Model file for the job. Use its own axes, mm. A direction names the side the tool comes from. Round coordinates to 2 decimals unless told otherwise and drop trailing zeros. Loops run counter-clockwise (first coordinate to the right, second up) from the corner with the lowest first, then second, coordinate; pieces in that order, holes last. Notation, with made-up numbers: M 67,20 L 108,20 A23 cw 108,37 Z; hole C -27,-18 d1. An arc over 180 degrees is marked long. Answer in a Markdown table with one row per item.
from build123d import *
from build123d.topology import SkipClean

# Parameters (mm, degrees)
SKETCH2_W                = 120
SKETCH2_H                = 250
BOSS_EXTRUDE1_DEPTH      = 50
CUT_EXTRUDE1_DEPTH       = 295.78805946
CUT_EXTRUDE1_DEPTH_BACK  = 295.78805946
CUT_EXTRUDE2_DEPTH       = 100
CUT_EXTRUDE3_DEPTH       = 282.780056072
CUT_EXTRUDE3_DEPTH_BACK  = 282.780056072
FILLET1_R                = 25
CUT_EXTRUDE5_DEPTH       = 60
FILLET4_R                = 12
SKETCH8_R                = 25
BOSS_EXTRUDE2_DEPTH      = 150.7
CUT_EXTRUDE11_DEPTH      = 422.260596306
CUT_EXTRUDE11_DEPTH_BACK = 422.260596306
SKETCH9_R                = 25


with BuildPart() as part:
    # Sketch2 → Boss-Extrude1 (new, symmetric)
    with BuildSketch(Plane(origin=(0, 0, 0), x_dir=(1, 0, 0), z_dir=(0, 1, 0))):
        with Locations((-60, 125)):
            Rectangle(SKETCH2_W, SKETCH2_H)
    extrude(amount=BOSS_EXTRUDE1_DEPTH, both=True)

    # Sketch3 → Cut-Extrude1 (cut, two sides: drawn at the far end of the back side and taken through both)
    with BuildSketch(Plane(origin=(0, 50, 0), x_dir=(1, 0, 0), z_dir=(0, 1, 0)).offset(-CUT_EXTRUDE1_DEPTH_BACK)):
        with BuildLine():
            Line((-120, 250), (-120, 104))
            ThreePointArc((-120, 104), (-115.759222637, 126.156468376), (-103.636363636, 145.180915101))
            ThreePointArc((-103.636363636, 145.180915101), (-93.533981136, 161.034620706), (-90, 179.498344353))
            Line((-90, 179.498344353), (-90, 250))
            Line((-90, 250), (-120, 250))
        make_face()
        with BuildLine():
            ThreePointArc((-16.363636364, 145.180915101), (-4.240777363, 126.156468376), (0, 104))
            Line((0, 104), (0, 250))
            Line((0, 250), (-30, 250))
            Line((-30, 250), (-30, 179.498344353))
            ThreePointArc((-30, 179.498344353), (-26.466018864, 161.034620706), (-16.363636364, 145.180915101))
        make_face()
        with BuildLine():
            ThreePointArc((-30, 100), (-38.786796564, 121.213203436), (-60, 130))
            Line((-60, 130), (-60, 0))
            Line((-60, 0), (-30, 0))
            Line((-30, 0), (-30, 100))
        make_face()
        with BuildLine():
            Line((-60, 0), (-60, 130))
            ThreePointArc((-60, 130), (-81.213203436, 121.213203436), (-90, 100))
            Line((-90, 100), (-90, 0))
            Line((-90, 0), (-60, 0))
        make_face()
    extrude(amount=CUT_EXTRUDE1_DEPTH + CUT_EXTRUDE1_DEPTH_BACK, mode=Mode.SUBTRACT)

    # Sketch4 → Cut-Extrude2 (cut)
    with BuildSketch(Plane(origin=(0, 0, 0), x_dir=(0, 0, -1), z_dir=(1, 0, 0))):
        Polygon((104, 50), (104, 29.703239367), (250, 29.703239367), (250, 50), (179.498344353, 50), (145.180915101, 50), align=None)
        Polygon((250, -30.296760633), (104, -30.296760633), (104, -50), (145.180915101, -50), (179.498344353, -50), (250, -50), align=None)
        with BuildLine():
            Line((104, -30.296760633), (89.331663554, -30.296760633))
            ThreePointArc((89.331663554, -30.296760633), (71.831443345, -44.802429848), (49.703239367, -50))
            Line((49.703239367, -50), (104, -50))
            Line((104, -50), (104, -30.296760633))
        make_face()
        with BuildLine():
            Line((89.331663554, 29.703239367), (104, 29.703239367))
            Line((104, 29.703239367), (104, 50))
            Line((104, 50), (0, 50))
            Line((0, 50), (0, -0.29676067))
            ThreePointArc((0, -0.29676067), (33.879981934, 46.820502952), (89.331663554, 29.703239367))
        make_face()
        with BuildLine():
            Line((0, -50), (49.703239367, -50))
            ThreePointArc((49.703239367, -50), (14.557741777, -35.442258249), (0, -0.29676067))
            Line((0, -0.29676067), (0, -50))
        make_face()
    extrude(amount=-CUT_EXTRUDE2_DEPTH, mode=Mode.SUBTRACT)

    # Sketch5 → Cut-Extrude3 (cut, two sides: drawn at the far end of the back side and taken through both)
    with SkipClean():  # the faces are left unmerged after this step: merging them gives an invalid solid
        with BuildSketch(Plane(origin=(0, 0, 0), x_dir=(0, 0, -1), z_dir=(1, 0, 0)).offset(-CUT_EXTRUDE3_DEPTH_BACK)):
            with BuildLine():
                Line((104, 29.703239367), (145.180915101, 29.703239367))
                Line((145.180915101, 29.703239367), (149.498344353, 29.703239367))
                Line((149.498344353, 29.703239367), (149.498344353, 50))
                Line((149.498344353, 50), (0, 50))
                Line((0, 50), (0, -0.296760633))
                ThreePointArc((0, -0.296760633), (33.879981952, 46.820502958), (89.331663554, 29.703239367))
                Line((89.331663554, 29.703239367), (104, 29.703239367))
            make_face()
            with BuildLine():
                ThreePointArc((49.703239367, -50), (14.557741764, -35.442258236), (0, -0.296760633))
                Line((0, -0.296760633), (0, -50))
                Line((0, -50), (49.703239367, -50))
            make_face()
            with BuildLine():
                Line((149.498344353, -30.296760633), (104, -30.296760633))
                Line((104, -30.296760633), (89.331663554, -30.296760633))
                ThreePointArc((89.331663554, -30.296760633), (71.831443345, -44.802429848), (49.703239367, -50))
                Line((49.703239367, -50), (149.498344353, -50))
                Line((149.498344353, -50), (149.498344353, -30.296760633))
            make_face()
        extrude(amount=CUT_EXTRUDE3_DEPTH + CUT_EXTRUDE3_DEPTH_BACK, mode=Mode.SUBTRACT)

    # Fillet1
    # the kernel refuses this fillet: 25 mm, written as the material it adds along each edge
    with BuildSketch(Plane(origin=(0, 29.703239367, -89.331663554), x_dir=(0, 0, -1), z_dir=(-1, 0, 0))) as fillet1_piece_1:
        with BuildLine():
            CenterArc((10.924260924, -25), FILLET1_R, 90, 42.587349398)
            Line((-5.993574748, -6.593837006), (-6.331931462, -6.225713746))
            ThreePointArc((-6.331931462, -6.225713746), (-3.218715087, -3.095193721), (-0.398650316, 0.301791195))
            Line((-0.398650316, 0.301791195), (0, 0.5))
            Line((0, 0.5), (10.924260924, 0.5))
            Line((10.924260924, 0.5), (10.924260924, 0))
        make_face()
    extrude(amount=30)
    with BuildSketch(Plane(origin=(-120, 29.703239367, -89.331663554), x_dir=(0, 0, -1), z_dir=(1, 0, 0)), Plane(origin=(-100, -30.296760633, -89.331663554), x_dir=(0, 0, -1), z_dir=(-1, 0, 0))) as fillet1_piece_2:
        with BuildLine():
            CenterArc((10.924260924, 25), FILLET1_R, 227.412650602, 42.587349398)
            Line((-5.993574748, 6.593837006), (-6.331931462, 6.225713746))
            ThreePointArc((-6.331931462, 6.225713746), (-3.218715087, 3.095193721), (-0.398650316, -0.301791195))
            Line((-0.398650316, -0.301791195), (0, -0.5))
            Line((0, -0.5), (10.924260924, -0.5))
            Line((10.924260924, -0.5), (10.924260924, 0))
        make_face()
    extrude(amount=20)
    with BuildSketch(Plane(origin=(0, -30.296760633, -89.331663554), x_dir=(0, -0.739986016552033, 0.6726222530569846), z_dir=(-1, 0, 0))) as fillet1_piece_3:
        with BuildLine():
            CenterArc((11.151749418, -24.899356651), FILLET1_R, 95.142875011, 42.587349398)
            Line((-7.347900995, -8.083800325), (-7.717894004, -7.747489198))
            Line((-7.717894004, -7.747489198), (-0.369993008, 0.336311127))
            Line((-0.369993008, 0.336311127), (0.04481981, 0.497987133))
            ThreePointArc((0.04481981, 0.497987133), (4.455379465, 0.299907981), (8.865939121, 0.497987133))
            Line((8.865939121, 0.497987133), (8.910758931, 0))
        make_face()
    extrude(amount=30)
    with BuildSketch(Plane(origin=(-90, -30.296760633, -89.331663554), x_dir=(0, 0, -1), z_dir=(-1, 0, 0))) as fillet1_piece_4:
        with BuildLine():
            CenterArc((10.924260924, 25), FILLET1_R, 227.412650602, 42.587349398)
            Line((-5.993574748, 6.593837006), (-6.331931462, 6.225713746))
            ThreePointArc((-6.331931462, 6.225713746), (-3.218715087, 3.095193721), (-0.398650316, -0.301791195))
            Line((-0.398650316, -0.301791195), (0, -0.5))
            Line((0, -0.5), (10.924260924, -0.5))
            Line((10.924260924, -0.5), (10.924260924, 0))
        make_face()
    extrude(amount=10)
    with BuildSketch(Plane(origin=(-90, 29.703239367, -89.331663554), x_dir=(0, 0, -1), z_dir=(-1, 0, 0))) as fillet1_piece_5:
        with BuildLine():
            CenterArc((10.924260924, -25), FILLET1_R, 90, 42.587349398)
            Line((-5.993574748, -6.593837006), (-6.331931462, -6.225713746))
            ThreePointArc((-6.331931462, -6.225713746), (-3.218715087, -3.095193721), (-0.398650316, 0.301791195))
            Line((-0.398650316, 0.301791195), (0, 0.5))
            Line((0, 0.5), (10.924260924, 0.5))
            Line((10.924260924, 0.5), (10.924260924, 0))
        make_face()
    extrude(amount=10)

    # Sketch6 → Cut-Extrude5 (cut)
    with BuildSketch(Plane(origin=(0, 0, -250), x_dir=(-1, 0, 0), z_dir=(0, 0, -1))):
        Polygon((30, 12.203239367), (47.5, 29.703239367), (30, 29.703239367), align=None)
        Polygon((90, 12.203239367), (90, 29.703239367), (72.5, 29.703239367), align=None)
        Polygon((90, -12.796760633), (72.5, -30.296760633), (90, -30.296760633), align=None)
        Polygon((47.5, -30.296760633), (30, -12.796760633), (30, -30.296760633), align=None)
    extrude(amount=-CUT_EXTRUDE5_DEPTH, mode=Mode.SUBTRACT)

    # Fillet4
    fillet4_edges = [part.edges().sort_by_distance(p)[0] for p in [
        (-38.75, -21.546760633, -190),
        (-81.25, -21.546760633, -190),
        (-81.25, 20.953239367, -190),
        (-38.75, 20.953239367, -190),
    ]]
    fillet(fillet4_edges, radius=FILLET4_R)

    # Sketch8 → Boss-Extrude2 (add)
    with BuildSketch(Plane(origin=(0, 0, -250), x_dir=(-1, 0, 0), z_dir=(0, 0, -1))):
        with Locations((60, -0.296760633)):
            Circle(SKETCH8_R)
    extrude(amount=BOSS_EXTRUDE2_DEPTH)

    # Sketch9 → Cut-Extrude11 (cut, two sides: drawn at the far end of the back side and taken through both)
    with BuildSketch(Plane.ZY.offset(120).offset(-CUT_EXTRUDE11_DEPTH_BACK)):
        with Locations((-46.609873597, -0.035297833)):
            Circle(SKETCH9_R)
    extrude(amount=CUT_EXTRUDE11_DEPTH + CUT_EXTRUDE11_DEPTH_BACK, mode=Mode.SUBTRACT)


solid = part.part
1. Tool access for faces 1 (the flat face through (-59, 29.703, -157)), 2 (the flat face through (-90, -1, -73)), 3 (the flat face through (-81.128, 21.076, -226.336)): list every direction of +Z, -Z, +X, -X, +Y, -Y with a clear straight run to the whole face (end or side of a thin tool).
Verdict:
| item | result |
|---|---|
| face 1 | -Z, +X, -X, +Y |
| face 2 | +Z, +Y, -Y |
| face 3 | -Z, -X, +Y |
2. Saw through at A-A (y = 5). Write the cut outline in (x, z), and give its area (3 significant figures).
Verdict:
| item | result |
|---|---|
| outline | M -120,-104 A60 ccw -103.64,-145.18 A50 cw -90,-179.5 L -90,-250 L -84.43,-250 L -84.43,-400.7 L -35.57,-400.7 L -35.57,-250 L -30,-250 L -30,-179.5 A50 cw -16.36,-145.18 A60 ccw 0,-104 L 0,-71.1 L -30,-71.1 L -30,-100 A30 cw -90,-100 L -90,-71.1 L -120,-71.1 Z; M -120,-22.12 L -90,-22.12 L -90,-0.28 L -120,-0.28 Z; M -30,-22.12 L 0,-22.12 L 0,-0.28 L -30,-0.28 Z |
| area | 20,600 mm² |
3. Saw through at C-C (z = -61.5). Write the cut outline in (x, y).
Verdict:
| item | result |
|---|---|
| outline | M -120,-48.58 L -90,-48.58 L -90,-20.12 L -120,-20.12 Z; M -120,20.05 L -90,20.05 L -90,47.99 L -120,47.99 Z; M -30,-48.58 L 0,-48.58 L 0,-20.12 L -30,-20.12 Z; M -30,20.05 L 0,20.05 L 0,47.99 L -30,47.99 Z |
4. Saw through at B-B (x = -95). Write the cut outline in (y, z).
Verdict:
| item | result |
|---|---|
| outline | M -36.89,-83.34 A25 cw -30.3,-100.26 L -30.3,-157.7 L 29.7,-157.7 L 29.7,-100.26 A25 cw 36.3,-83.34 A49.7 ccw long Z; hole C -0.04,-46.61 d50 |
5. Wall check: probe 1 along X at (y, z) = (22.5, -58); probe 2 along Y at (x, z) = (-66, -204); probe 3 along Z at (x, y) = (-15.5, -22.5). Give the ranges that are in metal, low to high.
Verdict:
| item | result |
|---|---|
| probe 1 | x = -120 to -90, -30 to 0 |
| probe 2 | y = -30.3 to 29.7 |
| probe 3 | z = -144.25 to -57.58, -35.64 to -5.23 |
6. Saw through at D-D (z = -228). Write the cut outline in (x, y).
Verdict:
| item | result |
|---|---|
| outline | M -90,-12.8 L -72.5,-30.3 L -47.5,-30.3 L -30,-12.8 L -30,12.2 L -47.5,29.7 L -72.5,29.7 L -90,12.2 Z |
7. Pin check, flat tips, straight feed: pin 1 (1 mm diameter, centred on x = -55.5, y = -24, fed in from +Z); pin 2 (1 mm diameter, centred on y = -7, z = -225, fed in from +X); pin 3 (6 mm diameter, centred on x = -80.5, y = 21.5, fed in from -Z). Stop position of each tip, or through.
Verdict:
| item | result |
|---|---|
| pin 1 | stops at z = -129.58 |
| pin 2 | stops at x = -30 |
| pin 3 | stops at z = -250 |
8. Mould opens along X. For faces 4 (the cylindrical face through (-104.79, 31.363, -91.299)), 5 (the flat face through (0, 0, -73)), 6 (the flat face through (-30, -26, -47)) say: +X half, -X half, draft (parallel to the pull), parting line (faces both ways), or undercut.
Verdict:
| item | result |
|---|---|
| face 4 | draft |
| face 5 | +X half |
| face 6 | undercut |
